Input: part model. Units: mm. Frame: model coordinates. Face numbers are marked on the shaded views. A direction names the side the tool comes from. Give positions to 0.01 mm unless a question says otherwise; leave off trailing zeros. Loops run counter-clockwise (first coordinate to the right, second up) from the corner with the lowest first, then second, coordinate; pieces in that order, holes last. Notation, with made-up numbers: (0.5, 22.25) - (20.5, 22.25) arc R15 ccw to (20.5, 37.25) - close; hole circle Ø9 at (32.25, 87.25). An arc over 180 degrees is marked (long way). Answer as a JSON object with one key per item and string values. Group by question number.
(1) Section query C-C (x = 4.5). Return loops of the section in (y, z).
(2) Mould query, pull axis Z, two halves, no side actions, for the marked faces 1, 2 and 3. Classes: +Z half, -Z half, draft (parallel to the pull), parting line (faces both ways), or undercut.
(3) Pin query (flat end, axial travel): P1, Ø5, axis at x = 6, y = 7.5, coming from the -Z side; P2, Ø6, axis at x = 7, z = -5, coming from the +Y side; P3, Ø1.5, axis at x = -10.5, y = 3, coming from the -Z side; P4, Ø6.5, axis at y = 2.5, z = -1, coming from the +X side. Return the tip coordinate at first contact, or that it passes through.
(4) Section query D-D (x = -16). Return loops of the section in (y, z).
(5) Material intervals for L1, parallel to Y at x = 8.5, z = 0; L2, parallel to Y at x = -12, z = -3.5; L3, parallel to X at y = -7.25, z = -7.25, sorted ascending.
(6) Access query for the marked faces 4 and 5. Directions: +Z, -Z, +X, -X, +Y, -Y. A direction counts if a zero-diameter tool reaches every point of the face in a straight line with its end or side. Return the directions, or none.
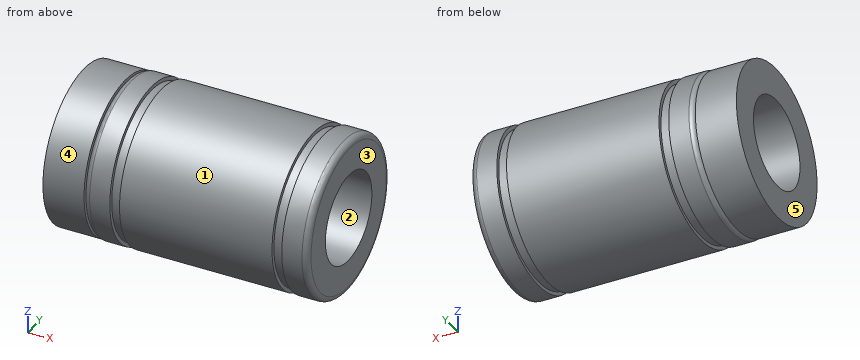
```python
from build123d import *

# Parameters (mm, degrees)
SKETCH2_W = 5.5
SKETCH2_H = 4.4


with BuildPart() as part:
    # Sketch1 → Revolve1 (revolve)
    with BuildSketch(Plane.XY, mode=Mode.PRIVATE) as revolve1_sk:
        with BuildLine():
            Line((-15, 9.7), (-15, 6))
            Line((-15, 6), (15, 6))
            Line((15, 6), (15, 9.7))
            ThreePointArc((15, 9.7), (14.765685425, 10.265685425), (14.2, 10.5))
            Line((14.2, 10.5), (11.5, 10.5))
            Line((11.5, 10.5), (11.5, 10))
            Line((11.5, 10), (10.2, 10))
            Line((10.2, 10), (10.2, 10.5))
            Line((10.2, 10.5), (-10.2, 10.5))
            Line((-10.2, 10.5), (-10.2, 10))
            Line((-10.2, 10), (-11.5, 10))
            Line((-11.5, 10), (-11.5, 10.5))
            Line((-11.5, 10.5), (-14.2, 10.5))
            ThreePointArc((-14.2, 10.5), (-14.765685425, 10.265685425), (-15, 9.7))
        make_face()
    revolve(revolve1_sk.sketch.rotate(Axis((15, 0, 0), (-1, 0, 0)), 270), axis=Axis((15, 0, 0), (-1, 0, 0)))

    # Sketch2 → Revolve2 (revolve)
    with BuildSketch(Plane.XY, mode=Mode.PRIVATE) as revolve2_sk:
        with Locations((-17.75, 8.2)):
            Rectangle(SKETCH2_W, SKETCH2_H)
    revolve(revolve2_sk.sketch.rotate(Axis((-15, 0, 0), (-1, 0, 0)), 270), axis=Axis((-15, 0, 0), (-1, 0, 0)))


solid = part.part
```
Recorded:
{
 "1": {"outline": "circle Ø21 at (0, 0); hole circle Ø12 at (0, 0)"},
 "2": {"face 1": "parting line", "face 2": "undercut", "face 3": "draft"},
 "3": {"P1": "stops at z = -9.23", "P2": "stops at y = 10.31", "P3": "stops at z = -10.24", "P4": "passes through"},
 "4": {"outline": "circle Ø20.8 at (0, 0); hole circle Ø12 at (0, 0)"},
 "5": {"L1": "y = -10.5 to -6, 6 to 10.5", "L2": "y = -9.9 to -4.87, 4.87 to 9.9", "L3": "x = -20.5 to -15, -14.78 to -11.5, -10.2 to 10.2, 11.5 to 14.78"},
 "6": {"face 4": "-X", "face 5": "+Z, -Z, -X, +Y, -Y"}
}
